```python
from build123d import *

# Parameters (mm, degrees)
SKETCH012_W                     = 85
SKETCH012_H                     = 50
PAD009_DEPTH                    = 17
SKETCH013_W                     = 14.870205
SKETCH013_H                     = 31.25
POCKET002_DEPTH                 = 11
POCKET003_DEPTH                 = 15
SKETCH018_W                     = 21.5
SKETCH018_H                     = 17
POCKET007_DEPTH                 = 16
CYLINDER002_R                   = 2.25
CYLINDER002_DEPTH               = 12
CYLINDER002_MIRRORED009_2_R     = 2.25
CYLINDER002_MIRRORED009_2_DEPTH = 12
SKETCH037_W                     = 24
SKETCH037_H                     = 17
POCKET014_DEPTH                 = 17.001
CHAMFER003_SIZE                 = 1.5


with BuildPart() as part:
    # Sketch012 → Pad009 (new body)
    with BuildSketch(Plane.XY):
        Rectangle(SKETCH012_W, SKETCH012_H)
    extrude(amount=PAD009_DEPTH)

    # Sketch013 → Pocket002 (cut)
    with BuildSketch(Plane.XY):
        with Locations((-39.027907, -0.625)):
            Rectangle(SKETCH013_W, SKETCH013_H)
    extrude(amount=POCKET002_DEPTH, mode=Mode.SUBTRACT)

    # Sketch014 → Pocket003 (cut)
    with BuildSketch(Plane.XY):
        Polygon((-33.474945, 23.25), (34, 23.25), (34, 16), (40.75, 16), (40.75, -16), (34, -16), (34, -23.25), (-33.474945, -23.25), align=None)
    extrude(amount=POCKET003_DEPTH, mode=Mode.SUBTRACT)

    # Sketch018 → Pocket007 (cut)
    with BuildSketch(Plane.XY):
        with Locations((-19.75, -13)):
            Rectangle(SKETCH018_W, SKETCH018_H)
    extrude(amount=POCKET007_DEPTH, mode=Mode.SUBTRACT)

    # Cylinder002 → Cylinder002 (cut)
    with BuildSketch(Plane(origin=(-37, 19.5, 0), x_dir=(1, 0, 0), z_dir=(0, 0, 1))):
        Circle(CYLINDER002_R)
    cylinder002 = extrude(amount=CYLINDER002_DEPTH, mode=Mode.SUBTRACT)

    # Cylinder002 Mirrored009 2 → Cylinder002 Mirrored009 2 (cut)
    with BuildSketch(Plane(origin=(37, 19.5, 0), x_dir=(-1, 0, 0), z_dir=(0, 0, -1))):
        Circle(CYLINDER002_MIRRORED009_2_R)
    cylinder002_mirrored009_2 = extrude(amount=-CYLINDER002_MIRRORED009_2_DEPTH, mode=Mode.SUBTRACT)

    # Mirrored010: Cylinder002, Cylinder002 Mirrored009 2 across XZ
    add(cylinder002.mirror(Plane.XZ), mode=Mode.SUBTRACT)
    add(cylinder002_mirrored009_2.mirror(Plane.XZ), mode=Mode.SUBTRACT)

    # Sketch037 → Pocket014 (cut, through all)
    with BuildSketch(Plane.XY):
        with Locations((22, 6)):
            Rectangle(SKETCH037_W, SKETCH037_H)
    extrude(amount=POCKET014_DEPTH, mode=Mode.SUBTRACT)

    # Chamfer003
    chamfer003_edges = [part.edges().sort_by_distance(p)[0] for p in [
        (22, 14.5, 17),
    ]]
    chamfer(chamfer003_edges, length=CHAMFER003_SIZE)


solid = part.part
```
Work out the finished part from the listing and answer in its coordinate system (mm). A direction names the side the tool comes from. Give positions to 0.01 mm unless a question says otherwise; leave off trailing zeros. Write each loop counter-clockwise with the first axis right and the second up, starting at its lowest first coordinate (ties: lowest second). Pieces come first, ordered by that corner, then holes. Notation, with made-up numbers: (-2.5, -14) -> (33.5, -14) arc R18 ccw to (33.5, -2) -> close; hole circle Ø1 at (73.25, 8). An arc over 180 degrees is marked (long way). Write item = value, one per line.
Q1. Section B-B on z = 6.5 is taken. Determine the outline of the cut face in (x, y).
Computed values:
outline = (-42.5, -25) -> (42.5, -25) -> (42.5, 25) -> (-42.5, 25) -> (-42.5, 15) -> (-33.47, 15) -> (-33.47, 23.25) -> (34, 23.25) -> (34, 16) -> (40.75, 16) -> (40.75, -16) -> (34, -16) -> (34, -23.25) -> (-33.47, -23.25) -> (-33.47, -16.25) -> (-42.5, -16.25) -> close; hole circle Ø4.5 at (-37, -19.5); hole circle Ø4.5 at (-37, 19.5); hole circle Ø4.5 at (37, -19.5); hole circle Ø4.5 at (37, 19.5)
Q2. For a pull along X with two mould halves and no side action, classify faces 1 (the flat face through (34, -20, 7)), 2 (the flat face through (-1, 0, 17)) as pulls with the +X half, pulls with the -X half, needs draft (parallel to the pull), parting line crosses it, or undercut.
Computed values:
face_1 = undercut
face_2 = needs draft
Q3. Flat-ended cylindrical pins translate along their axes: pin 1 Ø2.5 at (x, y) = (37, 19.5) entering from -Z; pin 2 Ø12 at (x, y) = (21.5, 10) entering from -Z; pin 3 Ø1 at (y, z) = (7, 5.5) entering from -X. Find the tip coordinate at first contact, or state that the pin passes through.
Computed values:
pin_1 = 12
pin_2 = 15
pin_3 = 40.75
Q4. Section D-D on y = 19.5 is taken. Determine the outline of the cut face in (x, z), and give its area (3 significant figures).
Computed values:
outline = (-42.5, 0) -> (-39.25, 0) -> (-39.25, 12) -> (-34.75, 12) -> (-34.75, 0) -> (-33.47, 0) -> (-33.47, 15) -> (34, 15) -> (34, 0) -> (34.75, 0) -> (34.75, 12) -> (39.25, 12) -> (39.25, 0) -> (42.5, 0) -> (42.5, 17) -> (-42.5, 17) -> close
area = 325 mm^2
Q5. Section C-C on x = -27.5 is taken. Determine the outline of the cut face in (y, z), and give its area (4 significant figures).
Computed values:
outline = (-25, 0) -> (-23.25, 0) -> (-23.25, 15) -> (-21.5, 15) -> (-21.5, 16) -> (-4.5, 16) -> (-4.5, 15) -> (23.25, 15) -> (23.25, 0) -> (25, 0) -> (25, 17) -> (-25, 17) -> close
area = 135.5 mm^2
Q6. Consider line 1 along X through (y, z) = (-19.5, 8.75); line 2 along Y through (x, z) = (37, 8); line 3 along Y through (x, z) = (-37, 4.5). Determine where each line is inside the solid, lowest interval first.
Computed values:
line_1 = -42.5 to -39.25, -34.75 to -33.47, 34 to 34.75, 39.25 to 42.5
line_2 = -25 to -21.75, -17.25 to -16, 16 to 17.25, 21.75 to 25
line_3 = -25 to -21.75, -17.25 to -16.25, 15 to 17.25, 21.75 to 25
Q7. Section A-A on y = -1.5 is taken. Determine the outline of the cut face in (x, z), and give its area (3 significant figures).
Computed values:
outline = (-42.5, 11) -> (-33.47, 11) -> (-33.47, 15) -> (10, 15) -> (10, 17) -> (-42.5, 17) -> close; (34, 15) -> (40.75, 15) -> (40.75, 0) -> (42.5, 0) -> (42.5, 17) -> (34, 17) -> close
area = 184 mm^2
Q8. A tool of negligible diameter and unlimited length cuts with its end or side. For faces 3 (the flat face through (37, 20, 12)), 4 (the flat face through (-38, 0, 11)), 5 (the flat face through (22, -2.5, 16)), from which of +Z, -Z, +X, -X, +Y, -Y can it reach the whole face along a straight path? Write none if from no direction.
Computed values:
face_3 = -Z
face_4 = -Z, -X
face_5 = +Z, -Z
